```python
from build123d import *

# Parameters (mm, degrees)
PAD_DEPTH            = 15
SKETCH001_W          = 7
SKETCH001_H          = 20
POCKET_DEPTH         = 97.489094
POCKET_DEPTH_BACK    = 97.489094
SKETCH002_R          = 1.5
POCKET001_DEPTH      = 109.489094
POCKET001_DEPTH_BACK = 109.489094
PAD001_DEPTH         = 10
SKETCH004_R          = 1.5
POCKET002_DEPTH      = 107.817154


with BuildPart() as part:
    # Sketch (on DatumPlane) → Pad (new body, symmetric)
    with BuildSketch(Plane.XZ):
        with BuildLine():
            ThreePointArc((-15, 3), (-18, 0), (-15, -3))
            Line((-15, -3), (15, -3))
            ThreePointArc((15, -3), (18, 0), (15, 3))
            Line((-15, 3), (15, 3))
        make_face()
    extrude(amount=PAD_DEPTH, both=True)

    # Sketch001 (on DatumPlane) → Pocket (cut, two sides)
    with BuildSketch(Plane.XY) as pocket_sk:
        with Locations((-14.5, 0)):
            Rectangle(SKETCH001_W, SKETCH001_H)
    pocket = extrude(amount=-POCKET_DEPTH, mode=Mode.SUBTRACT) + extrude(pocket_sk.sketch, amount=POCKET_DEPTH_BACK, mode=Mode.SUBTRACT)

    # Mirrored: Pocket across YZ
    add(pocket.mirror(Plane.YZ), mode=Mode.SUBTRACT)

    # Sketch002 (on DatumPlane) → Pocket001 (cut, two sides)
    with BuildSketch(Plane.XZ) as pocket001_sk:
        with Locations((-15, 0)):
            Circle(SKETCH002_R)
    pocket001 = extrude(amount=-POCKET001_DEPTH, mode=Mode.SUBTRACT) + extrude(pocket001_sk.sketch, amount=POCKET001_DEPTH_BACK, mode=Mode.SUBTRACT)

    # Mirrored001: Pocket001 across YZ
    add(pocket001.mirror(Plane.YZ), mode=Mode.SUBTRACT)

    # Sketch003 (on DatumPlane) → Pad001 (join)
    with BuildSketch(Plane.XZ.offset(5)):
        with BuildLine():
            Line((4, 8), (4, 3))
            Line((4, 3), (10, 3))
            Line((10, 3), (10, 8))
            ThreePointArc((10, 8), (7, 11), (4, 8))
        make_face()
    pad001 = extrude(amount=PAD001_DEPTH)

    # Sketch004 (on DatumPlane) → Pocket002 (cut, through all)
    with BuildSketch(Plane.XZ.offset(5)):
        with Locations((7, 8)):
            Circle(SKETCH004_R)
    pocket002 = extrude(amount=POCKET002_DEPTH, mode=Mode.SUBTRACT)

    # Mirrored002: Pad001, Pocket002 across XZ
    add(pad001.mirror(Plane.XZ))
    add(pocket002.mirror(Plane.XZ), mode=Mode.SUBTRACT)


solid = part.part
```
Can you work these out from the model? Positions are in its coordinate system, mm. A direction names the side the tool comes from. Round coordinates to 2 decimals unless told otherwise and drop trailing zeros. Order: outer loops, then holes, each group sorted by start corner. A loop starts at its lowest first (then second) coordinate and runs counter-clockwise, first axis right, second up. Notation, with made-up numbers: (44.5, 73) -> (67.5, 73) arc R13 cw to (67.5, 94) -> close; hole circle Ø5 at (21.25, 84.25). An arc over 180 degrees is marked (long way). Return JSON: item names as keys, results as strings. Group by question number.
1. Will these pins go through, and if not, where does the flat tip stop? pin 1 (5.5 mm diameter, centred on y = 11, z = 5, fed in from -X); pin 2 (2.5 mm diameter, centred on y = -8.5, z = 4.5, fed in from -X); pin 3 (1.5 mm diameter, centred on y = 10.5, z = 4.5, fed in from +X).
2. If we section it at B-B, the plane x = 7: Write out the boundary of the cut face in (y, z).
3. If we section it at D-D, the plane x = -13: Write out the boundary of the cut face in (y, z), then the cut area to 3 significant figures.
4. We'd pull the mould along Z, two halves only. Please class faces 1 (the face through (13, -10, 0)), 2 (the face through (-18, 12, 0)), 3 (the face through (5.8, 9.9, 7.1)), 4 (the face through (16.5, -12.54, 0.07)): released by +Z, released by -Z, zero draft, split by the parting line, or undercut.
5. Which directions (+Z, -Z, +X, -X, +Y, -Y) give clear straight access to the entire face, cutting with the end or side of a thin tool? Please do faces 5 (the face through (-13, 10, 0)), 6 (the face through (7, 5, 6)), 7 (the face through (13, 10, 0)).
6. If we section it at A-A, the plane z = 0: Write out the boundary of the cut face in (x, y).
7. I need wall thicknesses on line 1 (X direction, y = -11.8, z = 0); line 2 (Z direction, x = 15, y = -12.15); line 3 (Y direction, x = -15.5, z = 2.5). Which ranges of each line are inside material? Lowest first, please. Write a range as [from, to].
8. If we section it at C-C, the plane y = -12.5: Write out the boundary of the cut face in (x, z).
Output values:
{
 "1": {"pin 1": "x = -16.98", "pin 2": "x = 4", "pin 3": "x = 10"},
 "2": {"outline": "(-15, -3) -> (15, -3) -> (15, 6.5) -> (5, 6.5) -> (5, 3) -> (-5, 3) -> (-5, 6.5) -> (-15, 6.5) -> close; (-15, 9.5) -> (-5, 9.5) -> (-5, 11) -> (-15, 11) -> close; (5, 9.5) -> (15, 9.5) -> (15, 11) -> (5, 11) -> close"},
 "3": {"outline": "(-15, -3) -> (-10, -3) -> (-10, 3) -> (-15, 3) -> close; (10, -3) -> (15, -3) -> (15, 3) -> (10, 3) -> close", "area": "60.0 mm²"},
 "4": {"face 1": "zero draft", "face 2": "split by the parting line", "face 3": "undercut", "face 4": "undercut"},
 "5": {"face 5": "+Z, -Z, -X", "face 6": "+Z, +X, -X", "face 7": "+Z, -Z, +X"},
 "6": {"outline": "(-18, -15) -> (-16.5, -15) -> (-16.5, -10) -> (-18, -10) -> close; (-18, 10) -> (-16.5, 10) -> (-16.5, 15) -> (-18, 15) -> close; (-13.5, -15) -> (13.5, -15) -> (13.5, -10) -> (11, -10) -> (11, 10) -> (13.5, 10) -> (13.5, 15) -> (-13.5, 15) -> (-13.5, 10) -> (-11, 10) -> (-11, -10) -> (-13.5, -10) -> close; (16.5, -15) -> (18, -15) -> (18, -10) -> (16.5, -10) -> close; (16.5, 10) -> (18, 10) -> (18, 15) -> (16.5, 15) -> close"},
 "7": {"line 1": "[-18, -16.5], [-13.5, 13.5], [16.5, 18]", "line 2": "[-3, -1.5], [1.5, 3]", "line 3": "[-15, -10], [10, 15]"},
 "8": {"outline": "(-15, -3) -> (15, -3) arc R3 ccw to (15, 3) -> (10, 3) -> (10, 8) arc R3 ccw to (4, 8) -> (4, 3) -> (-15, 3) arc R3 ccw to start; hole circle Ø3 at (-15, 0); hole circle Ø3 at (7, 8); hole circle Ø3 at (15, 0)"}
}
